Build history of the part. All positions in model axes, mm. A direction names the side the tool comes from. Give positions to 0.01 mm unless a question says otherwise; leave off trailing zeros. Loops run counter-clockwise (first coordinate to the right, second up) from the corner with the lowest first, then second, coordinate; pieces in that order, holes last. Notation, with made-up numbers: (-7.5, 71.25) -> (1.5, 71.25) arc R21 cw to (1.5, 96.25) -> close; hole circle Ø8 at (85, 82.25). An arc over 180 degrees is marked (long way). Answer as a JSON object with one key per item and string values. Group by question number.
Q1. Band-saw the part on B-B, the plane x = 26. Write the cut outline in (y, z).
Q2. Band-saw the part on D-D, the plane z = -17.5. Write the cut outline in (x, y) (3 decimals).
Q3. Tool access for faces 1 (the flat face through (25, 1, 15)), 2 (the flat face through (19.094, -7.057, -33.592)), 3 (the flat face through (19, 0, 0)): list every direction of +Z, -Z, +X, -X, +Y, -Y with a clear straight run to the whole face (end or side of a thin tool).
Q4. Two-plate mould, pull along Y, no slides. Class faces 4 (the cylindrical face through (25.35, 2.26, 23.92)), 5 (the flat face through (20, -9, 32)), 6 (the flat face through (20, 1, 0)), 7 (the cylindrical face through (6.17, -3.41, -28.21)): pulls with the +Y half, pulls with the -Y half, needs draft (parallel to the pull), parting line crosses it, or undercut.
Q5. Band-saw the part on A-A, the plane z = 6. Write the cut outline in (x, y), plus the area to 3 significant figures.
Q6. Drop flat-ended pins along their axis: pin 1 (8 mm diameter, centred on x = 10.5, y = -7, fed in from +Z); pin 2 (4 mm diameter, centred on x = 34.5, z = -0.5, fed in from -Y); pin 3 (8 mm diameter, centred on x = 16.5, z = -27, fed in from +Y). Give the stop position or say it passes through.
Q7. Wall check: probe 1 along X at (y, z) = (1.15, 17.5) (3 decimals); probe 2 along X at (y, z) = (1.75, -6.5); probe 3 along Z at (x, y) = (44, -6.25). Give the ranges that are in metal, low to high. Write a range as from..to.
Q8. Band-saw the part on C-C, the plane y = -8.5. Write the cut outline in (x, z), plus the area to 3 significant figures.
from build123d import *

# Parameters (mm, degrees)
SKETCH1_W                      = 50
SKETCH1_H                      = 46
BASE_FLANGE1_DEPTH             = 2.5
EDGE_FLANGE1_STRIP_CUT_DEPTH   = 50
EDGE_FLANGE1_STRIP_CUT_2_DEPTH = 50
EDGE_FLANGE1_DEPTH             = 50
EDGE_FLANGE1_BEND_DEPTH        = 50
CUT_EXTRUDE1_REACH             = 83.004
SKETCH13_R                     = 1.875
CUT_EXTRUDE2_REACH             = 70.62
SKETCH14_R                     = 1.875
CHAMFER1_SIZE                  = 20
CUT_EXTRUDE3_REACH             = 70.62
SKETCH15_W                     = 10
SKETCH15_H                     = 30


# Sheet-metal steps are written as plain solids
with BuildPart() as part:
    # Sketch1 → Base-Flange1 (new body)
    with BuildSketch(Plane(origin=(0, 0, 0), x_dir=(1, 0, 0), z_dir=(0, 1, 0))):
        with Locations((25, 0)):
            Rectangle(SKETCH1_W, SKETCH1_H)
    extrude(amount=BASE_FLANGE1_DEPTH)

    # Edge-Flange1 strip (across the edge) → Edge-Flange1 strip cut (cut)
    with BuildSketch(Plane(origin=(0, 0, -23), x_dir=(0, -0.7071067811865512, 0.7071067811865438), z_dir=(1, 0, 0))):
        Polygon((-9.66479933, 6.129265424), (-1.552021808, -1.983512098), (0.215745145, -0.215745145), (-7.897032377, 7.897032377), align=None)
    extrude(amount=EDGE_FLANGE1_STRIP_CUT_DEPTH, mode=Mode.SUBTRACT)

    # Edge-Flange1 strip 2 (across the edge) → Edge-Flange1 strip cut 2 (cut)
    with BuildSketch(Plane(origin=(50, 0, 23), x_dir=(0, -0.7071067811865512, -0.7071067811865438), z_dir=(-1, 0, 0))):
        Polygon((-9.66479933, 6.129265424), (-1.552021808, -1.983512098), (0.215745145, -0.215745145), (-7.897032377, 7.897032377), align=None)
    extrude(amount=EDGE_FLANGE1_STRIP_CUT_2_DEPTH, mode=Mode.SUBTRACT)

    # Edge-Flange1 section (across the edge) → Edge-Flange1 (add)
    with BuildSketch(Plane(origin=(0, 0, -23), x_dir=(0, -0.7071067811865512, 0.7071067811865438), z_dir=(1, 0, 0))):
        with BuildLine():
            Line((-2.5, 0.30510971), (-2.5, 25))
            Line((-2.5, 25), (0, 25))
            Line((0, 25), (0, 0.30510971))
            ThreePointArc((0, 0.30510971), (0.056070336, 0.023225094), (0.215745145, -0.215745145))
            Line((0.215745145, -0.215745145), (-1.552021808, -1.983512098))
            ThreePointArc((-1.552021808, -1.983512098), (-2.253628495, -0.933483487), (-2.5, 0.30510971))
        make_face()
    extrude(amount=EDGE_FLANGE1_DEPTH)

    # Edge-Flange1 section 2 (across the edge) → Edge-Flange1 bend (add)
    with BuildSketch(Plane(origin=(50, 0, 23), x_dir=(0, -0.7071067811865512, -0.7071067811865438), z_dir=(-1, 0, 0))):
        with BuildLine():
            Line((-2.5, 0.30510971), (-2.5, 25))
            Line((-2.5, 25), (0, 25))
            Line((0, 25), (0, 0.30510971))
            ThreePointArc((0, 0.30510971), (0.056070336, 0.023225094), (0.215745145, -0.215745145))
            Line((0.215745145, -0.215745145), (-1.552021808, -1.983512098))
            ThreePointArc((-1.552021808, -1.983512098), (-2.253628495, -0.933483487), (-2.5, 0.30510971))
        make_face()
    extrude(amount=EDGE_FLANGE1_BEND_DEPTH)

    # Sketch13 → Cut-Extrude1 (cut, up to next)
    with BuildSketch(Plane(origin=(0, 13.267766953, 13.267766953), x_dir=(1, 0, 0), z_dir=(0, 0.7071067811865513, 0.7071067811865438)), mode=Mode.PRIVATE) as cut_extrude1_sk1:
        with Locations(Location((8, -22.763455967, 0), (0, 0, 270))):
            Circle(SKETCH13_R)
    cut_extrude1_tool1 = extrude(cut_extrude1_sk1.sketch, amount=-CUT_EXTRUDE1_REACH, mode=Mode.PRIVATE) & part.part
    # Sketch13 → Cut-Extrude1 (cut, up to next)
    with BuildSketch(Plane(origin=(0, 13.267766953, 13.267766953), x_dir=(1, 0, 0), z_dir=(0, 0.7071067811865513, 0.7071067811865438)), mode=Mode.PRIVATE) as cut_extrude1_sk2:
        with Locations(Location((8, -34.763455967, 0), (0, 0, 270))):
            Circle(SKETCH13_R)
    cut_extrude1_tool2 = extrude(cut_extrude1_sk2.sketch, amount=-CUT_EXTRUDE1_REACH, mode=Mode.PRIVATE) & part.part
    cut_extrude1_1 = cut_extrude1_tool1.solids().sort_by_distance((8, -2.828427, 29.363961))[0]
    add(cut_extrude1_1, mode=Mode.SUBTRACT)
    cut_extrude1_2 = cut_extrude1_tool2.solids().sort_by_distance((8, -11.313708, 37.849242))[0]
    add(cut_extrude1_2, mode=Mode.SUBTRACT)
    cut_extrude1 = cut_extrude1_1 + cut_extrude1_2  # Cut-Extrude1 as one shape, for the pattern or mirror that repeats it

    # Mirror1: Cut-Extrude1 across plane
    add(cut_extrude1.mirror(Plane.XY), mode=Mode.SUBTRACT)

    # Sketch14 → Cut-Extrude2 (cut, up to next)
    with BuildSketch(Plane(origin=(0, 2.5, 0), x_dir=(1, 0, 0), z_dir=(0, 1, 0)), mode=Mode.PRIVATE) as cut_extrude2_sk1:
        with Locations(Location((7.5, 17.5, 0), (0, 0, 270))):
            Circle(SKETCH14_R)
    cut_extrude2_tool1 = extrude(cut_extrude2_sk1.sketch, amount=-CUT_EXTRUDE2_REACH, mode=Mode.PRIVATE) & part.part
    # Sketch14 → Cut-Extrude2 (cut, up to next)
    with BuildSketch(Plane(origin=(0, 2.5, 0), x_dir=(1, 0, 0), z_dir=(0, 1, 0)), mode=Mode.PRIVATE) as cut_extrude2_sk2:
        with Locations(Location((42.5, 17.5, 0), (0, 0, 270))):
            Circle(SKETCH14_R)
    cut_extrude2_tool2 = extrude(cut_extrude2_sk2.sketch, amount=-CUT_EXTRUDE2_REACH, mode=Mode.PRIVATE) & part.part
    # Sketch14 → Cut-Extrude2 (cut, up to next)
    with BuildSketch(Plane(origin=(0, 2.5, 0), x_dir=(1, 0, 0), z_dir=(0, 1, 0)), mode=Mode.PRIVATE) as cut_extrude2_sk3:
        with Locations(Location((7.5, -17.5, 0), (0, 0, 270))):
            Circle(SKETCH14_R)
    cut_extrude2_tool3 = extrude(cut_extrude2_sk3.sketch, amount=-CUT_EXTRUDE2_REACH, mode=Mode.PRIVATE) & part.part
    # Sketch14 → Cut-Extrude2 (cut, up to next)
    with BuildSketch(Plane(origin=(0, 2.5, 0), x_dir=(1, 0, 0), z_dir=(0, 1, 0)), mode=Mode.PRIVATE) as cut_extrude2_sk4:
        with Locations(Location((42.5, -17.5, 0), (0, 0, 270))):
            Circle(SKETCH14_R)
    cut_extrude2_tool4 = extrude(cut_extrude2_sk4.sketch, amount=-CUT_EXTRUDE2_REACH, mode=Mode.PRIVATE) & part.part
    add(cut_extrude2_tool1.solids().sort_by_distance((7.5, 2.5, -17.5))[0], mode=Mode.SUBTRACT)
    add(cut_extrude2_tool2.solids().sort_by_distance((42.5, 2.5, -17.5))[0], mode=Mode.SUBTRACT)
    add(cut_extrude2_tool3.solids().sort_by_distance((7.5, 2.5, 17.5))[0], mode=Mode.SUBTRACT)
    add(cut_extrude2_tool4.solids().sort_by_distance((42.5, 2.5, 17.5))[0], mode=Mode.SUBTRACT)

    # Chamfer1
    chamfer1_edges = [part.edges().sort_by_distance(p)[0] for p in [
        (50, -16.793786053, -41.561553006),
        (50, -16.793786053, 41.561553006),
    ]]
    chamfer(chamfer1_edges, length=CHAMFER1_SIZE)

    # Sketch15 → Cut-Extrude3 (cut, up to next)
    with BuildSketch(Plane(origin=(0, 2.5, 0), x_dir=(1, 0, 0), z_dir=(0, 1, 0)), mode=Mode.PRIVATE) as cut_extrude3_sk1:
        with Locations((25, 0)):
            Rectangle(SKETCH15_W, SKETCH15_H)
    cut_extrude3_tool1 = extrude(cut_extrude3_sk1.sketch, amount=-CUT_EXTRUDE3_REACH, mode=Mode.PRIVATE) & part.part
    add(cut_extrude3_tool1.solids().sort_by_distance((25, 2.5, 0))[0], mode=Mode.SUBTRACT)


solid = part.part
Worked answers:
{
 "1": {"outline": "(-17.68, -40.68) -> (-15.91, -42.45) -> (1.55, -24.98) arc R3.24 ccw to (2.5, -22.69) -> (2.5, -15) -> (0, -15) -> (0, -22.69) arc R0.74 cw to (-0.22, -23.22) -> close; (-17.68, 40.68) -> (-0.22, 23.22) arc R0.74 cw to (0, 22.69) -> (0, 15) -> (2.5, 15) -> (2.5, 22.69) arc R3.24 ccw to (1.55, 24.98) -> (-15.91, 42.45) -> close"},
 "2": {"outline": "(0, 0) -> (5.625, 0) -> (5.625, 2.5) -> (0, 2.5) -> close; (9.375, 0) -> (40.625, 0) -> (40.625, 2.5) -> (9.375, 2.5) -> close; (44.375, 0) -> (50, 0) -> (50, 2.5) -> (44.375, 2.5) -> close"},
 "3": {"face 1": "+Y, -Y", "face 2": "-Z, +X, -X, +Y", "face 3": "+X, -X, -Y"},
 "4": {"face 4": "pulls with the +Y half", "face 5": "pulls with the -Y half", "face 6": "needs draft", "face 7": "undercut"},
 "5": {"outline": "(0, 0) -> (20, 0) -> (20, 2.5) -> (0, 2.5) -> close; (30, 0) -> (50, 0) -> (50, 2.5) -> (30, 2.5) -> close", "area": "100 mm2"},
 "6": {"pin 1": "z = 37.54", "pin 2": "y = 0", "pin 3": "y = 2.49"},
 "7": {"probe 1": "0..5.625, 9.375..40.625, 44.375..50", "probe 2": "0..20, 30..50", "probe 3": "-32.31..-29.25, 29.25..32.31"},
 "8": {"outline": "(0, -35.04) -> (40.48, -35.04) -> (42.98, -31.5) -> (0, -31.5) -> close; (0, 31.5) -> (42.98, 31.5) -> (40.48, 35.04) -> (0, 35.04) -> close", "area": "295 mm2"}
}
